from build123d import *

# Parameters (mm, degrees)
BOSS_EXTRUDE1_DEPTH = 5
SKETCH2_W           = 70
SKETCH2_H           = 50
BOSS_EXTRUDE2_DEPTH = 35
SKETCH3_W           = 40
SKETCH3_H           = 30
BOSS_EXTRUDE3_DEPTH = 30
SKETCH4_R           = 5
BOSS_EXTRUDE4_DEPTH = 5
SKETCH5_R           = 30
BOSS_EXTRUDE5_DEPTH = 30
SKETCH6_R           = 7.5
BOSS_EXTRUDE6_DEPTH = 130
SKETCH7_R           = 25
BOSS_EXTRUDE7_DEPTH = 5
SKETCH9_R           = 10
BOSS_EXTRUDE8_DEPTH = 30
SKETCH10_W          = 97.144237238
SKETCH10_H          = 25.610753454
BOSS_EXTRUDE9_DEPTH = 20
SHELL1_START        = -105
SHELL1_OUTLINE_R    = 20
SHELL1_DEPTH        = 10
SHELL1_START_2      = 95
SHELL1_2_OUTLINE_R  = 20
SHELL1_2_DEPTH      = 10


# Read off the part's stored shape, not the designer's step: Shell1
with BuildPart() as part:
    # Sketch1 → Boss-Extrude1 (new body)
    with BuildSketch(Plane.XY):
        with BuildLine():
            Line((-98.994949366, 35), (-82.994949366, 35))
            Line((-82.994949366, 35), (-82.994949366, 0))
            Line((-82.994949366, 0), (-82.994949366, -35))
            Line((-82.994949366, -35), (-98.994949366, -35))
            ThreePointArc((-98.994949366, -35), (0, -105), (98.994949366, -35))
            Line((98.994949366, -35), (82.994949366, -35))
            Line((82.994949366, -35), (82.994949366, 0))
            Line((82.994949366, 0), (82.994949366, 35))
            Line((82.994949366, 35), (98.994949366, 35))
            ThreePointArc((98.994949366, 35), (0, 105), (-98.994949366, 35))
        make_face()
    extrude(amount=BOSS_EXTRUDE1_DEPTH)

    # Sketch2 → Boss-Extrude2 (add)
    with BuildSketch(Plane.XY.offset(5)):
        Rectangle(SKETCH2_W, SKETCH2_H)
    extrude(amount=BOSS_EXTRUDE2_DEPTH)

    # Sketch3 → Boss-Extrude3 (add)
    with BuildSketch(Plane.XY.offset(5)):
        with Locations((60, 0)):
            Rectangle(SKETCH3_W, SKETCH3_H)
    boss_extrude3 = extrude(amount=BOSS_EXTRUDE3_DEPTH)

    # Sketch4 → Boss-Extrude4 (add)
    with BuildSketch(Plane(origin=(80, 0, 0), x_dir=(0, 0, -1), z_dir=(1, 0, 0))):
        with Locations(Location((-20, 0, 0), (0, 0, 180))):
            Circle(SKETCH4_R)
    boss_extrude4 = extrude(amount=BOSS_EXTRUDE4_DEPTH)

    # Sketch5 → Boss-Extrude5 (add)
    with BuildSketch(Plane(origin=(85, 0, 0), x_dir=(0, 0, -1), z_dir=(1, 0, 0))):
        with Locations((-20, 0)):
            Circle(SKETCH5_R)
    boss_extrude5 = extrude(amount=BOSS_EXTRUDE5_DEPTH)

    # Mirror1: Boss-Extrude3, Boss-Extrude4, Boss-Extrude5 across plane
    add(boss_extrude3.mirror(Plane(origin=(0, 0, 0), x_dir=(0, 0, 1), z_dir=(1, 0, 0))))
    add(boss_extrude4.mirror(Plane(origin=(0, 0, 0), x_dir=(0, 0, 1), z_dir=(1, 0, 0))))
    add(boss_extrude5.mirror(Plane(origin=(0, 0, 0), x_dir=(0, 0, 1), z_dir=(1, 0, 0))))

    # Sketch6 → Boss-Extrude6 (add)
    with BuildSketch(Plane(origin=(0, 0, 0), x_dir=(-1, 0, 0), z_dir=(0, 0, -1))):
        with Locations(Location((0, 0, 0), (0, 0, 180))):
            Circle(SKETCH6_R)
    extrude(amount=BOSS_EXTRUDE6_DEPTH)

    # Sketch7 → Boss-Extrude7 (add)
    with BuildSketch(Plane(origin=(0, 0, -130), x_dir=(-1, 0, 0), z_dir=(0, 0, -1))):
        Circle(SKETCH7_R)
    extrude(amount=BOSS_EXTRUDE7_DEPTH)

    # Sketch9 → Boss-Extrude8 (add)
    with BuildSketch(Plane(origin=(0, 0, -135), x_dir=(-1, 0, 0), z_dir=(0, 0, -1))):
        with Locations((0, 14)):
            Circle(SKETCH9_R)
        with Locations((0, -14)):
            Circle(SKETCH9_R)
    extrude(amount=BOSS_EXTRUDE8_DEPTH)

    # Sketch10 → Boss-Extrude9 (add)
    with BuildSketch(Plane.XY.offset(5)):
        with Locations((0, 60)):
            Rectangle(SKETCH10_W, SKETCH10_H)
    boss_extrude9 = extrude(amount=BOSS_EXTRUDE9_DEPTH)

    # Mirror2: Boss-Extrude9 across plane
    add(boss_extrude9.mirror(Plane.ZX))

    # Shell1 outline → Shell1 (cut)
    with BuildSketch(Plane.YZ.offset(SHELL1_START)):
        with Locations((0, 20)):
            Circle(SHELL1_OUTLINE_R)
    extrude(amount=SHELL1_DEPTH, mode=Mode.SUBTRACT)

    # Shell1 2 outline → Shell1 2 (cut)
    with BuildSketch(Plane.YZ.offset(SHELL1_START_2)):
        with Locations((0, 20)):
            Circle(SHELL1_2_OUTLINE_R)
    extrude(amount=SHELL1_2_DEPTH, mode=Mode.SUBTRACT)


solid = part.part
Here's how the part is built. I have some questions about the finished solid (model axes, mm). A direction names the side the tool comes from. Give positions to 0.01 mm unless a question says otherwise; leave off trailing zeros. Loops run counter-clockwise (first coordinate to the right, second up) from the corner with the lowest first, then second, coordinate; pieces in that order, holes last. Notation, with made-up numbers: (-12, 5) -> (3, 5) arc R6 ccw to (3, 12) -> close; hole circle Ø10 at (-11.5, 55.5). An arc over 180 degrees is marked (long way). One line per item, written item: value.
Q1. I'm going to push flat-ended pins straight in: pin 1 Ø2.5 at (x, z) = (88, 3) entering from +Y; pin 2 Ø2.5 at (x, z) = (-87.5, 2) entering from +Y; pin 3 Ø5.5 at (x, z) = (-94, 3.5) entering from -Y. Where does each tip first touch, or does it pass through?
Answers follow:
pin 1: y = 59.16
pin 2: y = 59.88
pin 3: y = -51.95
Q2. Suppose I cut it at D-D on z = -142. Please give me the cut outline in (x, y), then the cut area to 3 significant figures.
Answers follow:
outline: circle Ø20 at (0, -14); circle Ø20 at (0, 14)
area: 628 mm^2
Q3. On a 3-axis mill with a long thin cutter (end or side, diameter ignored), from which of +Z, -Z, +X, -X, +Y, -Y can I reach the whole of each face in a straight line? I mean faces 1 (the face through (48.572, 60, 15)), 2 (the face through (-1, 47.195, 15)), 3 (the face through (-60, -15, 20)). Say none if no direction works.
Answers follow:
face 1: +Z, +X, +Y
face 2: +Z, +X, -X
face 3: +Z
Q4. Suppose I cut it at B-B on z = -5.5. Please give me the cut outline in (x, y), then the cut area to 3 significant figures.
Answers follow:
outline: (-115, -15.8) -> (-85, -15.8) -> (-85, 15.8) -> (-115, 15.8) -> close; circle Ø15 at (0, 0); (85, -15.8) -> (115, -15.8) -> (115, 15.8) -> (85, 15.8) -> close
area: 2,070 mm^2
Q5. We'd pull the mould along Y, two halves only. Please class faces 4 (the face through (35, 0, 22)), 5 (the face through (-1, -72.805, 15)), 6 (the face through (-48.572, 60, 15)): pulls with the +Y half, pulls with the -Y half, needs draft (parallel to the pull), parting line crosses it, or undercut.
Answers follow:
face 4: undercut
face 5: pulls with the -Y half
face 6: needs draft
Q6. If I drill on line 1 along Y through (x, z) = (-26, 13.5); line 2 along Y through (x, z) = (37.5, 13.5); line 3 along Z through (x, y) = (97, -15), over which ranges is the centre line in solid material (lowest first)?
Answers follow:
line 1: -72.81 to -47.19, -25 to 25, 47.19 to 72.81
line 2: -72.81 to -47.19, 47.19 to 72.81
line 3: -5.98 to 6.77, 33.23 to 45.98
Q7. Suppose I cut it at C-C on z = 20. State how many separate pieces and enclosed holes the cut face has, then the cut area to 3 significant figures.
Answers follow:
separate pieces: 5
enclosed holes: 2
area: 13,800 mm^2
Q8. Suppose I cut it at A-A on x = -17. Please give me the cut outline in (y, z).
Answers follow:
outline: (-103.61, 0) -> (103.61, 0) -> (103.61, 5) -> (72.81, 5) -> (72.81, 25) -> (47.19, 25) -> (47.19, 5) -> (25, 5) -> (25, 40) -> (-25, 40) -> (-25, 5) -> (-47.19, 5) -> (-47.19, 25) -> (-72.81, 25) -> (-72.81, 5) -> (-103.61, 5) -> close; (-18.33, -135) -> (18.33, -135) -> (18.33, -130) -> (-18.33, -130) -> close
